Job drawing, mm, ordinate dimensions from the low corner. One solid piece. A direction names the side the tool comes from. Give positions to 0.01 mm unless a question says otherwise; leave off trailing zeros. Order: outer loops, then holes, each group sorted by start corner. A loop starts at its lowest first (then second) coordinate and runs counter-clockwise, first axis right, second up. Notation, with made-up numbers: (52, 25) - (78, 25) arc R21 ccw to (78, 48) - close; hole circle Ø9 at (67.5, 63.25). An arc over 180 degrees is marked (long way). Use one line per item in the form item = value. Start each with the question number.
1. Drill centre line: line 1 (Z direction, x = 14, y = 4.65). Where is it in solid material? Low to high.
2. Band-saw the part on C-C, the plane y = 4.75. List the corners of the cut face in (x, z), plus the area to 3 significant figures.
3. Band-saw the part on A-A, the plane z = 22.5. List the corners of the cut face in (x, y).
4. Pin check, flat tips, straight feed: P1, Ø4, axis at x = 21, z = 21, coming from the -Y side; P2, Ø3, axis at x = 15.5, y = 3.5, coming from the -Z side. Stop position of each tip, or through.
5. Band-saw the part on B-B, the plane x = 12.25. List the corners of the cut face in (y, z), plus the area to 3 significant figures.
6. Pull direction X, two halves, no side cores. Call the marked faces 1, 2, 3 and 4: +X half, -X half, draft (parallel to the pull), parting line (faces both ways), or undercut.
7. Tool access for the marked faces 5 and 6: list every direction of +Z, -Z, +X, -X, +Y, -Y with a clear straight run to the whole face (end or side of a thin tool).
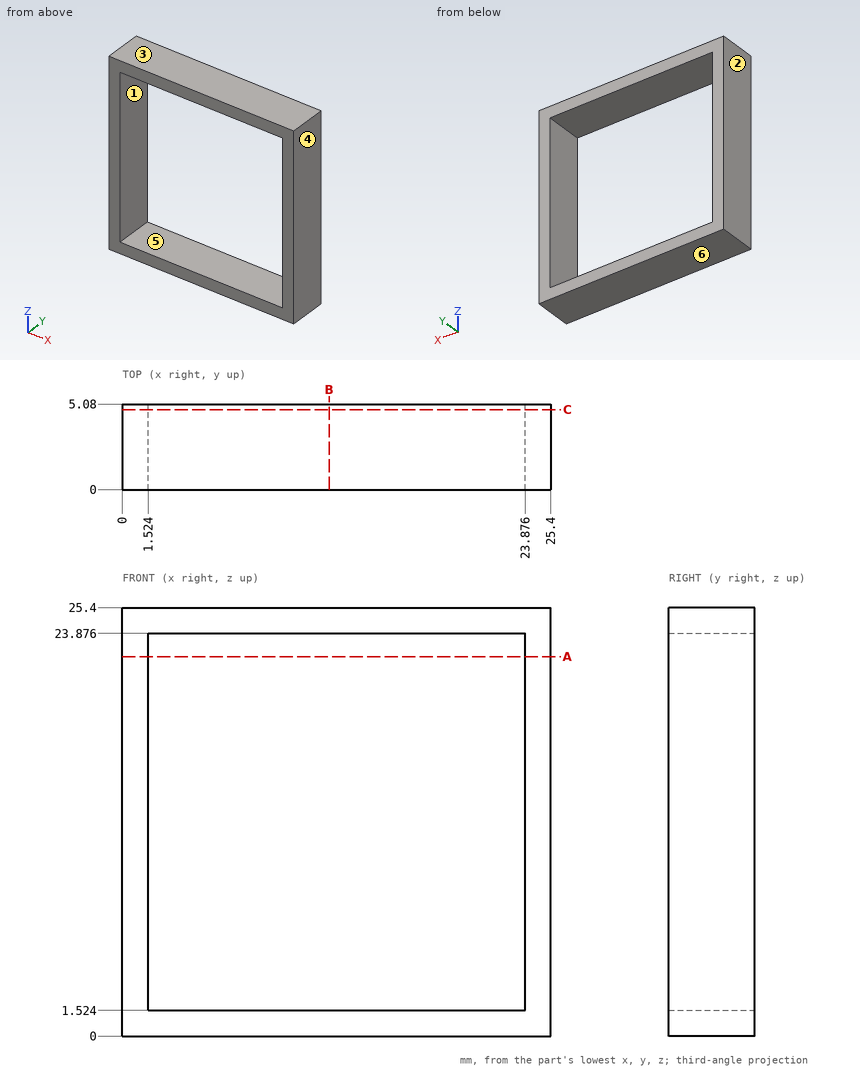
From the geometry:
q1.line_1 = 0 to 1.52, 23.88 to 25.4
q2.outline = (0, 0) - (25.4, 0) - (25.4, 25.4) - (0, 25.4) - close; hole (1.52, 1.52) - (23.88, 1.52) - (23.88, 23.88) - (1.52, 23.88) - close
q2.area = 146 mm²
q3.outline = (0, 0) - (1.52, 0) - (1.52, 5.08) - (0, 5.08) - close; (23.88, 0) - (25.4, 0) - (25.4, 5.08) - (23.88, 5.08) - close
q4.P1 = through
q4.P2 = 0
q5.outline = (0, 0) - (5.08, 0) - (5.08, 1.52) - (0, 1.52) - close; (0, 23.88) - (5.08, 23.88) - (5.08, 25.4) - (0, 25.4) - close
q5.area = 15.5 mm²
q6.face_1 = undercut
q6.face_2 = -X half
q6.face_3 = draft
q6.face_4 = +X half
q7.face_5 = +Y, -Y
q7.face_6 = -Z, +X, -X, +Y, -Y
